Model file for the job. Use its own axes, mm. Round coordinates to 2 decimals unless told otherwise and drop trailing zeros. Loops run counter-clockwise (first coordinate to the right, second up) from the corner with the lowest first, then second, coordinate; pieces in that order, holes last. Notation, with made-up numbers: M -2,52 L 14,52 A30 ccw 14,77 Z; hole C 72.25,-9.75 d1. An arc over 180 degrees is marked long. Use a Markdown table: item, result. Add a question column.
Q1. Cut at B-B (z = 0). Give the cut face in (x, y) (1 decimal).
Q2. Probe line 1 (Y direction, x = 25.5, z = -4.75); line 2 (Z direction, x = 4.25, y = 7); line 3 (X direction, y = 11, z = 0) (1 decimal). List the from-to ranges inside material, lowest first. Write a range as from..to.
Q3. Pin check, flat tips, straight feed: pin 1 (12 mm diameter, centred on x = 11.5, y = -8, fed in from -Z); pin 2 (12 mm diameter, centred on y = 6.5, z = -1.5, fed in from -X); pin 3 (5 mm diameter, centred on x = 15.5, z = 11.5, fed in from +Y). Stop position of each tip, or through.
Q4. Cut at D-D (x = 25.25). Give the cut face in (y, z) (1 decimal), plus the area to 3 significant figures.
Q5. Cut at A-A (y = 0). Give the cut face in (x, z) (1 decimal).
Q6. Mould opens along Z. For faces 1 (the face through (14.474, 0.628, 14.274)), 2 (the face through (28.575, -11, 3)), 3 (the face through (5.63, 9.82, -6.48)) say: +Z half, -Z half, draft (parallel to the pull), parting line (faces both ways), or undercut.
Q7. Cut at C-C (x = 14). Give the cut face in (y, z) (1 decimal), plus the area to 3 significant figures.
from build123d import *

# Parameters (mm, degrees)
SKETCH1_R           = 14.2875
SKETCH1_R_2         = 10.9093
BOSS_EXTRUDE1_DEPTH = 28.575
SKETCH2_R           = 9.5885
CUT_EXTRUDE1_DEPTH  = 19.05
CHAMFER1_SIZE       = 0.762


with BuildPart() as part:
    # Sketch1 → Boss-Extrude1 (new body)
    with BuildSketch(Plane(origin=(0, 0, 0), x_dir=(0, 0, -1), z_dir=(1, 0, 0))):
        Circle(SKETCH1_R)
        Circle(SKETCH1_R_2, mode=Mode.SUBTRACT)
    extrude(amount=BOSS_EXTRUDE1_DEPTH)

    # Sketch2 → Cut-Extrude1 (cut, symmetric)
    with BuildSketch(Plane(origin=(0, 0, 0), x_dir=(1, 0, 0), z_dir=(0, 1, 0))):
        with Locations((12.7, 0)):
            Circle(SKETCH2_R)
    extrude(amount=CUT_EXTRUDE1_DEPTH, both=True, mode=Mode.SUBTRACT)

    # Chamfer1
    chamfer1_edges = [part.edges().sort_by_distance(p)[0] for p in [
        (0, 0, 14.2875),
    ]]
    chamfer(chamfer1_edges, length=CHAMFER1_SIZE)


solid = part.part
Checked values:
| question | item | result |
|---|---|---|
| 1 | outline | M 0,-13.5 L 0.8,-14.3 L 3.1,-14.3 L 3.1,-10.9 L 0,-10.9 Z; M 0,10.9 L 3.1,10.9 L 3.1,14.3 L 0.8,14.3 L 0,13.5 Z; M 22.3,-14.3 L 28.6,-14.3 L 28.6,-10.9 L 22.3,-10.9 Z; M 22.3,10.9 L 28.6,10.9 L 28.6,14.3 L 22.3,14.3 Z |
| 2 | line 1 | y = -13.47..-9.82, 9.82..13.47 |
| 2 | line 2 | z = -12.46..-8.37, 8.37..12.46 |
| 2 | line 3 | x = 0..3.1, 22.3..28.6 |
| 3 | pin 1 | stops at z = -14.15 |
| 3 | pin 2 | stops at x = 0 |
| 3 | pin 3 | stops at y = 11.07 |
| 4 | outline | C 0,0 d28.6; hole C 0,0 d21.8 |
| 4 | area | 267 mm^2 |
| 5 | outline | M 0,-13.5 L 0.8,-14.3 L 28.6,-14.3 L 28.6,-10.9 L 0,-10.9 Z; M 0,10.9 L 28.6,10.9 L 28.6,14.3 L 0.8,14.3 L 0,13.5 Z |
| 6 | face 1 | parting line |
| 6 | face 2 | draft |
| 6 | face 3 | undercut |
| 7 | outline | M -10.7,-9.5 A14.3 ccw 10.7,-9.5 L 5.4,-9.5 A10.9 cw -5.4,-9.5 Z; M -10.7,9.5 L -5.4,9.5 A10.9 cw 5.4,9.5 L 10.7,9.5 A14.3 ccw Z |
| 7 | area | 121 mm^2 |
